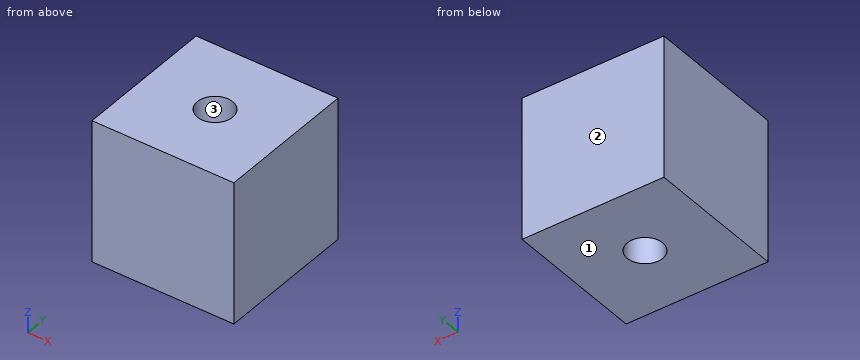
from build123d import *

# Parameters (mm, degrees)
SKETCH_1_W          = 60
SKETCH_1_H          = 60
EXTRUDE_1_DEPTH     = 30
SKETCH_2_R          = 7.5
CUT_EXTRUDE_1_DEPTH = 74.484692283


with BuildPart() as part:
    # 草图1 → 凸台-拉伸1 (new, symmetric)
    with BuildSketch(Plane.XY):
        Rectangle(SKETCH_1_W, SKETCH_1_H)
    extrude(amount=EXTRUDE_1_DEPTH, both=True)

    # 草图2 → 切除-拉伸1 (cut, through all)
    with BuildSketch(Plane(origin=(0, 0, 30), x_dir=(-1, 0, 0), z_dir=(0, 0, -1))):
        Circle(SKETCH_2_R)
    extrude(amount=CUT_EXTRUDE_1_DEPTH, mode=Mode.SUBTRACT)


solid = part.part
Geometry: final body of the model. Coordinates: model frame, mm. Face numbers are marked on the shaded views. Give positions to 0.01 mm unless a question says otherwise; leave off trailing zeros. Write each loop counter-clockwise with the first axis right and the second up, starting at its lowest first coordinate (ties: lowest second). Pieces come first, ordered by that corner, then holes.
(1) Cut plane C-C, the plane z = -17.5. Return loops of the section in (x, y), then the cut area to 3 significant figures.
(2) Ray query, line 1 (Y direction, x = 0, z = -8); line 2 (X direction, y = 4, z = -15). Return the intervals inside material, ascending.
(3) Cut plane A-A, the plane x = 0. Return loops of the section in (y, z), then the cut area to 3 significant figures.
(4) Mould query, pull axis Y, two halves, no side actions, for the marked faces 1, 2 and 3. Classes: released by +Y, released by -Y, zero draft, split by the parting line, or undercut.
Values follow:
1. outline: (-30, -30) - (30, -30) - (30, 30) - (-30, 30) - close; hole circle Ø15 at (0, 0)
1. area: 3,420 mm2
2. line 1: y = -30 to -7.5, 7.5 to 30
2. line 2: x = -30 to -6.34, 6.34 to 30
3. outline: (-30, -30) - (-7.5, -30) - (-7.5, 30) - (-30, 30) - close; (7.5, -30) - (30, -30) - (30, 30) - (7.5, 30) - close
3. area: 2,700 mm2
4. face 1: zero draft
4. face 2: released by +Y
4. face 3: undercut
